For this review, take the finished solid that the model builds, in its own axes (mm). A direction names the side the tool comes from. Give positions to 0.01 mm unless a question says otherwise; leave off trailing zeros. Loops run counter-clockwise (first coordinate to the right, second up) from the corner with the lowest first, then second, coordinate; pieces in that order, holes last. Notation, with made-up numbers: (63.5, 74.25) - (85.5, 74.25) arc R11 ccw to (85.5, 89.25) - close; hole circle Ø1 at (55.25, 54). An arc over 180 degrees is marked (long way). Put each result on its own line as item: value.
from build123d import *

# Parameters (mm, degrees)
F0_W     = 300
F0_H     = 300
F1_DEPTH = 9
F3_DEPTH = 300.001
F4_R     = 1.49999
F5_R     = 5.99999
F7_DEPTH = 300.001
F8_R     = 5.99999
F9_R     = 1.49999


# Not quite as in the source:
# - a fillet or chamfer is up to 0.001 mm smaller than in the source, because OpenCascade refuses the exact size


with BuildPart() as f1:
    # F0 (on Front) → F1 (new body, symmetric)
    with BuildSketch(Plane.XZ):
        with Locations((-3.7248600274, -5.7776198197)):
            Rectangle(F0_W, F0_H)
    extrude(amount=F1_DEPTH, both=True)

    # F2 (on face) → F3 (cut, through all)
    with BuildSketch(Plane.YZ.offset(146.2751399726)):
        Polygon((6, 144.2223801803), (-9, 144.2223801803), (-9, 127.2223801803), (-6, 127.2223801803), (-6, 119.2223801803), (6, 119.2223801803), align=None)
    extrude(amount=-F3_DEPTH, mode=Mode.SUBTRACT)

    # F4 (radius 1.5 in the source; OpenCascade refuses exactly that, so slightly less here)
    f4_edges = [f1.edges().sort_by_distance(p)[0] for p in [
        (-3.72486, 6, 144.22238),
        (-3.72486, 9, 144.22238),
        (-3.72486, -9, 127.22238),
        (-3.72486, -6, 127.22238),
    ]]
    fillet(f4_edges, radius=F4_R)

    # F5 (radius 6 in the source; OpenCascade refuses exactly that, so slightly less here)
    f5_edges = [f1.edges().sort_by_distance(p)[0] for p in [
        (-3.72486, 6, 119.22238),
        (-3.72486, -6, 119.22238),
    ]]
    fillet(f5_edges, radius=F5_R)

    # F6 (on face) → F7 (cut, through all)
    with BuildSketch(Plane(origin=(0, 0, -155.7776198197), x_dir=(1, 0, 0), z_dir=(0, 0, -1))):
        Polygon((146.2751399726, -6), (146.2751399726, 9), (129.2751399726, 9), (129.2751399726, 6), (121.2751399726, 6), (121.2751399726, -6), align=None)
    extrude(amount=-F7_DEPTH, mode=Mode.SUBTRACT)

    # F8 (radius 6 in the source; OpenCascade refuses exactly that, so slightly less here)
    f8_edges = [f1.edges().sort_by_distance(p)[0] for p in [
        (121.27514, 6, -15.277625),
        (121.27514, -6, -15.277625),
    ]]
    fillet(f8_edges, radius=F8_R)

    # F9 (radius 1.5 in the source; OpenCascade refuses exactly that, so slightly less here)
    f9_edges = [f1.edges().sort_by_distance(p)[0] for p in [
        (129.27514, -6, -15.027615),
        (146.27514, 9, -6.527615),
    ]]
    fillet(f9_edges, radius=F9_R)


solid = f1.part
1) For faces 1 (the face through (-15, -9, -13)), 2 (the face through (129, 6, 59)), list the 3-axis set-ups (+Z, -Z, +X, -X, +Y, -Y) from which the entire face can be reached by the end or side of a thin tool; tool diameter is ignored.
Geometry check:
face 1: +Z, -Z, +X, -X, -Y
face 2: +Z, +X
2) Wall thickness on line 1 (Z direction, x = -46, y = -7.25); line 2 (X direction, y = -0.25, z = -27.5); line 3 (Z direction, x = 76, y = 0.5): over which ranges is each line inside the solid? List them lowest first.
Geometry check:
line 1: z = -155.78 to 127.2
line 2: x = -153.72 to 121.28
line 3: z = -155.78 to 119.24
3) Insertion check: pin 1 Ø5 at (y, z) = (4.5, 11.5) entering from +X; pin 2 Ø5 at (y, z) = (-5.5, -92.5) entering from +X. Each pin has a flat end and moves straight along its axis. Give the tip position at first contact, or say it passes through.
Geometry check:
pin 1: stops at x = 146.19
pin 2: stops at x = 129.28
4) Take a section at C-C on y = -3. State the section outline as (x, z) points.
Geometry check:
outline: (-153.72, -155.78) - (122.08, -155.78) - (122.08, 120.03) - (-153.72, 120.03) - close
